from build123d import *

# Parameters (mm, degrees)
SKETCH1_R                   = 4
BOSS_EXTRUDE1_DEPTH         = 34
SKETCH2_R                   = 2
BOSS_EXTRUDE2_DEPTH         = 12
SKETCH3_W                   = 1.5
SKETCH3_H                   = 12
CUT_EXTRUDE1_DEPTH          = 5
CUT_EXTRUDE1_DEPTH_BACK     = 5
M3_TAPPED_HOLE1_D           = 2.5
M3_TAPPED_HOLE1_DEPTH       = 14
M3_TAPPED_HOLE1_CSINK_D     = 3.05
M3_TAPPED_HOLE1_CSINK_ANGLE = 90
M3_TAPPED_HOLE1_TIP         = 0.751075774
SKETCH7_R                   = 2
CUT_EXTRUDE2_DEPTH          = 12


with BuildPart() as part:
    # Sketch1 → Boss-Extrude1 (new body)
    with BuildSketch(Plane(origin=(0, 0, 0), x_dir=(1, 0, 0), z_dir=(0, 1, 0))):
        Circle(SKETCH1_R)
    extrude(amount=BOSS_EXTRUDE1_DEPTH)

    # Sketch2 → Boss-Extrude2 (add)
    with BuildSketch(Plane(origin=(0, 34, 0), x_dir=(1, 0, 0), z_dir=(0, 1, 0))):
        Circle(SKETCH2_R)
    extrude(amount=BOSS_EXTRUDE2_DEPTH)

    # Sketch3 → Cut-Extrude1 (cut, two sides)
    with BuildSketch(Plane.XY) as cut_extrude1_sk:
        with Locations((3.25, 15.5)):
            Rectangle(SKETCH3_W, SKETCH3_H)
    extrude(amount=CUT_EXTRUDE1_DEPTH, mode=Mode.SUBTRACT)
    extrude(cut_extrude1_sk.sketch, amount=-CUT_EXTRUDE1_DEPTH_BACK, mode=Mode.SUBTRACT)

    # M3 Tapped Hole1
    with Locations(Plane(origin=(0, 0, 0), x_dir=(-1, 0, 0), z_dir=(0, -1, 0))):
        with Locations((0, 0)):
            CounterSinkHole(M3_TAPPED_HOLE1_D / 2, M3_TAPPED_HOLE1_CSINK_D / 2, depth=M3_TAPPED_HOLE1_DEPTH, counter_sink_angle=M3_TAPPED_HOLE1_CSINK_ANGLE)
            with Locations((0, 0, -(M3_TAPPED_HOLE1_DEPTH + M3_TAPPED_HOLE1_TIP / 2))):  # 118° drill point
                Cone(0, M3_TAPPED_HOLE1_D / 2, M3_TAPPED_HOLE1_TIP, mode=Mode.SUBTRACT)

    # Sketch7 → Cut-Extrude2 (cut)
    with BuildSketch(Plane(origin=(0, 0, 0), x_dir=(0, 0, -1), z_dir=(1, 0, 0))):
        with Locations((0, 11.5)):
            Circle(SKETCH7_R)
    extrude(amount=-CUT_EXTRUDE2_DEPTH, mode=Mode.SUBTRACT)


solid = part.part
Check sheet for the modelled part. Datum: model origin and axes. Units: mm. A direction names the side the tool comes from. Give positions to 0.01 mm unless a question says otherwise; leave off trailing zeros. Loops run counter-clockwise (first coordinate to the right, second up) from the corner with the lowest first, then second, coordinate; pieces in that order, holes last. Notation, with made-up numbers: M 0.25,48 L 39.25,48 A28 cw 39.25,78 Z; hole C 41.5,-23 d1. An arc over 180 degrees is marked long. Return JSON: item names as keys, results as strings. Group by question number.
1. Cross-section at D-D on y = 37. Record the boundary of the cut face in (x, z).
2. Cross-section at A-A on z = 2.5. Record the boundary of the cut face in (x, y).
3. Thickness scan on L1, parallel to Y at x = -1.75, z = 0; L2, parallel to Z at x = 0, y = 8; L3, parallel to Y at x = 3.25, z = -2. Record the ranges inside material, lowest first.
4. Mould release check, pull along Z, two halves, no side actions. Record for faces 6 (the cylindrical face through (-4, 17, 0)), 7 (the cylindrical face through (1.19, 7.23, -0.38)), 8 (the flat face through (0, 46, 0)): released by +Z, released by -Z, zero draft, split by the parting line, or undercut.
5. Go/stop test with flat-tipped pins: pin 1 (2 mm diameter, centred on x = 3, y = 27, fed in from +Z); pin 2 (3 mm diameter, centred on x = 2.5, y = 16, fed in from -Z); pin 3 (0.6 mm diameter, centred on y = 11.5, z = -2, fed in from -X). Record where each tip stops, or that it passes through.
6. Cross-section at B-B on y = 11.5. Record the boundary of the cut face in (x, z), plus the area to 3 significant figures.
7. Tool access check on faces 1 (the cylindrical face through (0, 40, 2)), 2 (the flat face through (2, 0, 0)), 3 (the cylindrical face through (-1.972, 13.186, -1.075)), 4 (the conical face through (0.05, 14.62, 0.21)), 5 (the flat face through (3, 9.5, 0)). Record the directions out of +Z, -Z, +X, -X, +Y, -Y that give a thin tool (end or side, any length) a straight path to the whole face; none if there is none.
8. Cross-section at C-C on y = 24. Record the boundary of the cut face in (x, z), plus the area to 3 significant figures.
Return value:
{
 "1": {"outline": "C 0,0 d4"},
 "2": {"outline": "M -3.12,0 L 3.12,0 L 3.12,9.5 L 2.5,9.5 L 2.5,21.5 L 3.12,21.5 L 3.12,34 L -3.12,34 Z"},
 "3": {"L1": "0 to 9.5, 13.5 to 46", "L2": "-4 to -1.25, 1.25 to 4", "L3": "0 to 9.5, 21.5 to 34"},
 "4": {"face 6": "split by the parting line", "face 7": "undercut", "face 8": "zero draft"},
 "5": {"pin 1": "z = 3.46", "pin 2": "z = -3.87", "pin 3": "x = -3.48"},
 "6": {"outline": "M -3.46,-2 A4 ccw 2.5,-3.12 L 2.5,3.12 A4 ccw -3.46,2 L 0,2 L 0,1.25 A1.25 cw 0,-1.25 L 0,-2 Z", "area": "26.0 mm^2"},
 "7": {"face 1": "+Y", "face 2": "+Z, -Z, +X, -X, -Y", "face 3": "-X", "face 4": "-Y", "face 5": "+Z, -Z, +X"},
 "8": {"outline": "C 0,0 d8", "area": "50.3 mm^2"}
}
